Work out the finished part from the listing and answer in its coordinate system (mm). Face numbers are marked on the shaded views. A direction names the side the tool comes from. Coordinates: 2 decimals unless noted, no trailing zeros. Write each loop counter-clockwise with the first axis right and the second up, starting at its lowest first coordinate (ties: lowest second). Pieces come first, ordered by that corner, then holes. Notation, with made-up numbers: (83.5, 71) - (141.5, 71) arc R25 ccw to (141.5, 107) - close; hole circle Ø7 at (80.5, 24.25). An arc over 180 degrees is marked (long way). Use one line per item in the form item = value. Start each with the question number.
Item 1: A cutting plane is placed at A-A (y = 8). Write down the section's boundary in (x, z).
Item 2: Consider probe 1 along Y at (x, z) = (0, 13.75); probe 2 along Y at (x, z) = (1, -14); probe 3 along Y at (x, z) = (1, 3.5). Determine where each line is inside the solid, lowest interval first.
Item 3: A cutting plane is placed at D-D (y = -30.5). Write down the section's boundary in (x, z), then the cut area to 3 significant figures.
Item 4: For the marked faces 1 and 2, determine the directions among +Z, -Z, +X, -X, +Y, -Y from which every point of the face is accessible in a straight line to the end or side of a thin tool.
Item 5: Given pin 1 (2 mm diameter, centred on x = 4.5, y = -9.5, fed in from -Z); pin 2 (3.5 mm diameter, centred on y = 8, z = -14, fed in from -X); pin 3 (8 mm diameter, centred on x = 1.5, z = -12.5, fed in from -Y), each flat-ended and moving along its own axis, determine where each tip first touches the part or whether it passes through.
Item 6: A cutting plane is placed at B-B (z = -34). Write down the section's boundary in (x, y), then the cut area to 3 significant figures.
Item 7: A cutting plane is placed at C-C (x = -4.75). Write down the section's boundary in (y, z), then the cut area to 3 significant figures.
from build123d import *

# Parameters (mm, degrees)
BOSS_EXTRUDE1_DEPTH          = 8
SKETCH2_R                    = 3
CUT_EXTRUDE1_DEPTH           = 58.861904566
F_5_0_5_DIAMETER_HOLE2_D     = 5
F_5_0_5_DIAMETER_HOLE2_DEPTH = 12
F_5_0_5_DIAMETER_HOLE2_TIP   = 1.502151548


with BuildPart() as part:
    # Sketch1 → Boss-Extrude1 (new, symmetric)
    with BuildSketch(Plane(origin=(0, 0, 0), x_dir=(0, 0, -1), z_dir=(1, 0, 0))):
        Polygon((0, 0), (0, -34), (-16, -34), (-16, 16), (44, 16), (44, 0), align=None)
    extrude(amount=BOSS_EXTRUDE1_DEPTH, both=True)

    # Sketch2 → Cut-Extrude1 (cut, through all)
    with BuildSketch(Plane.ZY.offset(8)):
        with Locations((-34, 8)):
            Circle(SKETCH2_R)
        with Locations((-14, 8)):
            Circle(SKETCH2_R)
    extrude(amount=-CUT_EXTRUDE1_DEPTH, mode=Mode.SUBTRACT)

    # Ø5.0 (5) Diameter Hole2
    with Locations(Plane(origin=(0, 1, 16), x_dir=(1, 0, 0), z_dir=(0, 0, 1))):
        with Locations((0, 0), (0, -25)):
            Hole(F_5_0_5_DIAMETER_HOLE2_D / 2, depth=F_5_0_5_DIAMETER_HOLE2_DEPTH)
            with Locations((0, 0, -(F_5_0_5_DIAMETER_HOLE2_DEPTH + F_5_0_5_DIAMETER_HOLE2_TIP / 2))):  # 118° drill point
                Cone(0, F_5_0_5_DIAMETER_HOLE2_D / 2, F_5_0_5_DIAMETER_HOLE2_TIP, mode=Mode.SUBTRACT)


solid = part.part
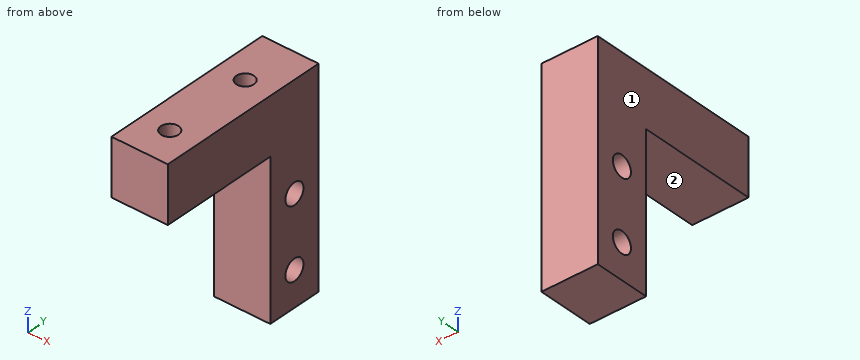
Answer:
q1.outline = (-8, -44) - (8, -44) - (8, -37) - (-8, -37) - close; (-8, -31) - (8, -31) - (8, -17) - (-8, -17) - close; (-8, -11) - (8, -11) - (8, 16) - (-8, 16) - close
q2.probe_1 = -34 to -26.5, -21.5 to -1.5, 3.5 to 16
q2.probe_2 = 0 to 5, 11 to 16
q2.probe_3 = -34 to -25.33, -22.67 to -0.33, 2.33 to 16
q3.outline = (-8, 0) - (8, 0) - (8, 16) - (-8, 16) - close
q3.area = 256 mm²
q4.face_1 = +Z, -Z, -X, +Y, -Y
q4.face_2 = -Z, +X, -X, -Y
q5.pin_1 = 0
q5.pin_2 = through
q5.pin_3 = 0
q6.outline = (-8, 0) - (8, 0) - (8, 5) - (-8, 5) - close; (-8, 11) - (8, 11) - (8, 16) - (-8, 16) - close
q6.area = 160 mm²
q7.outline = (-34, 0) - (0, 0) - (0, -44) - (16, -44) - (16, 16) - (-34, 16) - close; hole circle Ø6 at (8, -34); hole circle Ø6 at (8, -14)
q7.area = 1,450 mm²
